```python
from build123d import *

# Parameters (mm, degrees)
SKETCH_W        = 73.5
SKETCH_H        = 23.3
PAD_DEPTH       = 37
SKETCH001_W     = 67.5
SKETCH001_H     = 17.3
POCKET_DEPTH    = 34
SKETCH002_W     = 23.3
SKETCH002_H     = 6
PAD001_DEPTH    = 20
SKETCH003_R     = 1.5
POCKET001_DEPTH = 30


with BuildPart() as part:
    # Sketch → Pad (new body)
    with BuildSketch(Plane.XY):
        with Locations((2.379754, 0.114429)):
            Rectangle(SKETCH_W, SKETCH_H)
    extrude(amount=PAD_DEPTH)

    # Sketch001 (on Face6 of Pad) → Pocket (cut)
    with BuildSketch(Plane.XY.offset(37)):
        with Locations((2.379754, 0.114429)):
            Rectangle(SKETCH001_W, SKETCH001_H)
    extrude(amount=-POCKET_DEPTH, mode=Mode.SUBTRACT)

    # Sketch002 (on Face6 of Pocket) → Pad001 (join)
    with BuildSketch(Plane.YZ.offset(39.129754)):
        with Locations((0.114429, 34)):
            Rectangle(SKETCH002_W, SKETCH002_H)
    extrude(amount=PAD001_DEPTH)

    # Sketch003 (on Face4 of Pad001) → Pocket001 (cut)
    with BuildSketch(Plane(origin=(0, 0, 31), x_dir=(1, 0, 0), z_dir=(0, 0, -1))):
        with Locations((49.129754, -0.114429)):
            Circle(SKETCH003_R)
    extrude(amount=-POCKET001_DEPTH, mode=Mode.SUBTRACT)


solid = part.part
```
Geometry check sheet. Reference: the model listing, model coordinates, mm. A direction names the side the tool comes from. Round coordinates to 2 decimals unless told otherwise and drop trailing zeros. Order: outer loops, then holes, each group sorted by start corner. A loop starts at its lowest first (then second) coordinate and runs counter-clockwise, first axis right, second up. Notation, with made-up numbers: (18.25, 70.25) -> (28.25, 70.25) arc R5 ccw to (28.25, 74.25) -> close; hole circle Ø6 at (64, 33.5). An arc over 180 degrees is marked (long way). Return JSON: item names as keys, results as strings. Group by question number.
Q1. Section check A-A, the plane x = 48.5. Record the boundary of the cut face in (y, z), plus the area to 3 significant figures.
Q2. Release check for a two-part mould opening along Y. For faces 1 (the flat face through (2, -8.536, 20)), 2 (the flat face through (2, 0, 0)), 3 (the flat face through (1, 11.764, 18)), 4 (the flat face through (36.13, 0, 20)) record: released by +Y, released by -Y, zero draft, split by the parting line, or undercut.
Q3. Gauge pin test, flat ends, axial feed: pin 1 (8 mm diameter, centred on x = 42, z = 22, fed in from +Y); pin 2 (8.5 mm diameter, centred on y = 1.5, z = 20.5, fed in from +X); pin 3 (10 mm diameter, centred on x = 49.5, y = 2.5, fed in from -Z); pin 4 (8.5 mm diameter, centred on x = -12, y = -1, fed in from +Z). Record the tip position at first contact, or that the pin passes through.
Q4. Section check B-B, the plane y = -2.5. Record the boundary of the cut face in (x, z).
Q5. Tool access check on faces 5 (the flat face through (-31.37, 0, 20)), 6 (the flat face through (47, 0, 31)), 7 (the flat face through (1, -11.536, 18)). Record the directions out of +Z, -Z, +X, -X, +Y, -Y that give a thin tool (end or side, any length) a straight path to the whole face; none if there is none.
Q6. Material ranges on probe 1 along X at (y, z) = (2.25, 5.5); probe 2 along Y at (x, z) = (-28, 12.5); probe 3 along X at (y, z) = (-5.75, 2.5), recorded low to high. Write a range as from..to.
Q7. Section check D-D, the plane x = 31. Record the boundary of the cut face in (y, z), plus the area to 3 significant figures.
Q8. Section check C-C, the plane z = 9.5. Record the boundary of the cut face in (x, y).
Numbers:
{
 "1": {"outline": "(-11.54, 31) -> (-1.25, 31) -> (-1.25, 37) -> (-11.54, 37) -> close; (1.48, 31) -> (11.76, 31) -> (11.76, 37) -> (1.48, 37) -> close", "area": "123 mm^2"},
 "2": {"face 1": "undercut", "face 2": "zero draft", "face 3": "released by +Y", "face 4": "undercut"},
 "3": {"pin 1": "y = 11.76", "pin 2": "x = 39.13", "pin 3": "z = 31", "pin 4": "z = 3"},
 "4": {"outline": "(-34.37, 0) -> (39.13, 0) -> (39.13, 31) -> (59.13, 31) -> (59.13, 37) -> (36.13, 37) -> (36.13, 3) -> (-31.37, 3) -> (-31.37, 37) -> (-34.37, 37) -> close"},
 "5": {"face 5": "+Z", "face 6": "-Z, +X, +Y, -Y", "face 7": "+Z, -Z, +X, -X, -Y"},
 "6": {"probe 1": "-34.37..-31.37, 36.13..39.13", "probe 2": "-11.54..-8.54, 8.76..11.76", "probe 3": "-34.37..39.13"},
 "7": {"outline": "(-11.54, 0) -> (11.76, 0) -> (11.76, 37) -> (8.76, 37) -> (8.76, 3) -> (-8.54, 3) -> (-8.54, 37) -> (-11.54, 37) -> close", "area": "274 mm^2"},
 "8": {"outline": "(-34.37, -11.54) -> (39.13, -11.54) -> (39.13, 11.76) -> (-34.37, 11.76) -> close; hole (-31.37, -8.54) -> (36.13, -8.54) -> (36.13, 8.76) -> (-31.37, 8.76) -> close"}
}
